Drawing for the job (mm, zero at the part's lowest x, y, z). Coordinates: 2 decimals unless noted, no trailing zeros. Loops run counter-clockwise (first coordinate to the right, second up) from the corner with the lowest first, then second, coordinate; pieces in that order, holes last. Notation, with made-up numbers: (66, -31.5) -> (99, -31.5) arc R12 ccw to (99, -9.5) -> close; hole circle Ø3 at (-1.5, 50.5). An arc over 180 degrees is marked (long way). Write each question's results on one line, items separated by ' | '.
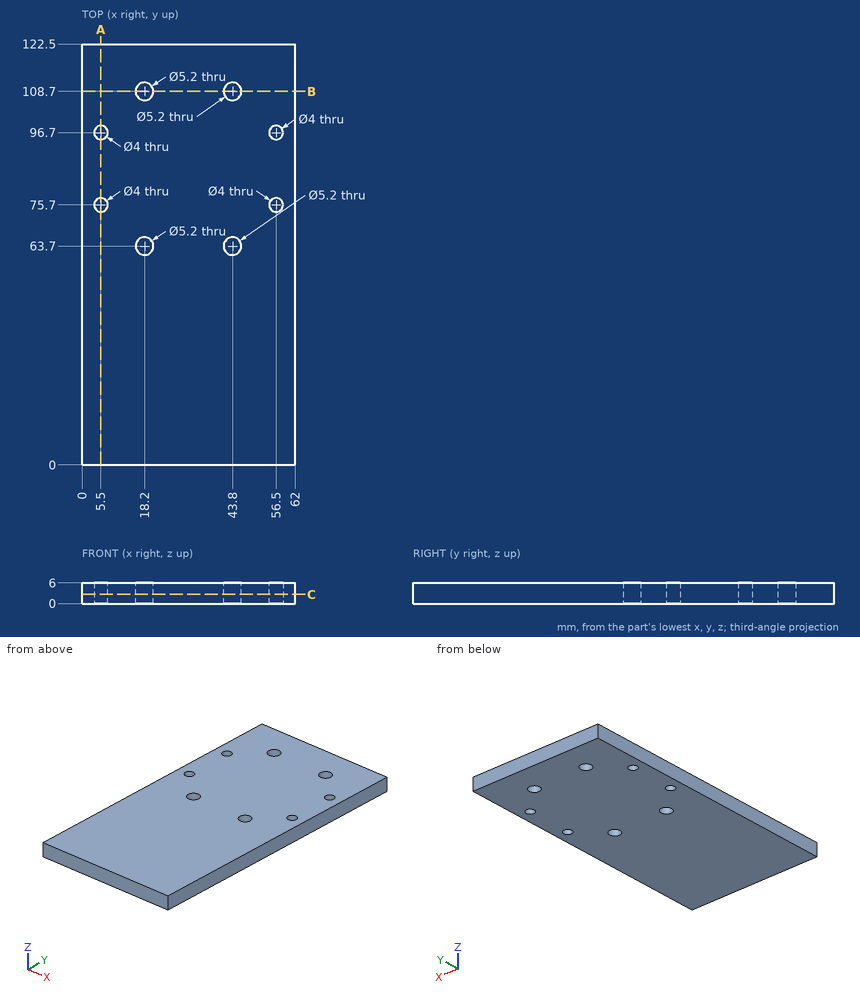
1) Slice it at B-B (y = 108.7). Write the cut outline in (x, z).
Outcome:
outline: (0, 0) -> (15.6, 0) -> (15.6, 6) -> (0, 6) -> close; (20.8, 0) -> (41.2, 0) -> (41.2, 6) -> (20.8, 6) -> close; (46.4, 0) -> (62, 0) -> (62, 6) -> (46.4, 6) -> close
2) Slice it at C-C (z = 2.7). Count the separate pieces of the cut face and the enclosed holes in it, then the cut area to 3 significant figures.
Outcome:
separate pieces: 1 | enclosed holes: 8 | area: 7,460 mm^2
3) Drill centre lines: L1, parallel to Y at x = 56.5, z = 4.35; L2, parallel to Y at x = 18.2, z = 1.4; L3, parallel to X at y = 75.7, z = 4.4. Where is each one in solid material? Low to high. Write a range as from..to.
Outcome:
L1: y = 0..73.7, 77.7..94.7, 98.7..122.5 | L2: y = 0..61.1, 66.3..106.1, 111.3..122.5 | L3: x = 0..3.5, 7.5..54.5, 58.5..62
4) Slice it at A-A (x = 5.5). Write the cut outline in (y, z), then the cut area to 3 significant figures.
Outcome:
outline: (0, 0) -> (73.7, 0) -> (73.7, 6) -> (0, 6) -> close; (77.7, 0) -> (94.7, 0) -> (94.7, 6) -> (77.7, 6) -> close; (98.7, 0) -> (122.5, 0) -> (122.5, 6) -> (98.7, 6) -> close | area: 687 mm^2
